Read the model definition and answer for the solid it produces. Units are mm, in the model's axes. A direction names the side the tool comes from. Give positions to 0.01 mm unless a question says otherwise; leave off trailing zeros. Write each loop counter-clockwise with the first axis right and the second up, starting at its lowest first coordinate (ties: lowest second). Pieces come first, ordered by that corner, then holes. Notation, with made-up numbers: (8.5, -10.5) -> (30.5, -10.5) arc R19 ccw to (30.5, 8.5) -> close; hole circle Ø9 at (-24, 65). An arc over 180 degrees is marked (long way). Answer as CSV lines item,"result". Start each with the question number.
1. Find the intervals of material crossed by line 1 (Y direction, x = 3, z = 78) (3 decimals); line 2 (Z direction, x = 1.5, y = 58.5) (3 decimals); line 3 (Y direction, x = 2.5, z = -12.5), in increasing order.
2. For a pull along Z with two mould halves and no side action, classify faces 3 (the cylindrical face through (3.219, 59.238, -17.206)), 4 (the flat face through (3, -43, -104.775)), 5 (the flat face through (3, -25, 53.975)), 6 (the flat face through (3, 69.85, 39)) as pulls with the +Z half, pulls with the -Z half, needs draft (parallel to the pull), parting line crosses it, or undercut.
3. The part is cut by section B-B, the plane y = -49. Determine the outline of the cut face in (x, z) (3 decimals).
4. The part is cut by section A-A, the plane x = 2.5. Give the number of separate pieces and of enclosed holes in the cut face, and give its area (3 significant figures).
5. A tool of negligible diameter and unlimited length cuts with its end or side. For faces 1 (the cylindrical face through (3.22, -103.11, 59.89)), 2 (the flat face through (3, 9.525, 80)), from which of +Z, -Z, +X, -X, +Y, -Y can it reach the whole face along a straight path? Write none if from no direction.
6. Given pin 1 (3 mm diameter, centred on y = 57.15, z = 60.325, fed in from +X); pin 2 (6.5 mm diameter, centred on y = 57.15, z = -15.875, fed in from +X); pin 3 (1.9 mm diameter, centred on x = 4, y = -13, fed in from +Z) (3 decimals); pin 4 (3 mm diameter, centred on x = 2.5, z = 67.5, fed in from +Y), each flat-ended and moving along its own axis, determine where each tip first touches the part or whether it passes through.
from build123d import *

# Parameters (mm, degrees)
SKETCH1_R               = 14.2875
BOSS_EXTRUDE1_DEPTH     = 6.35
SKETCH2_W               = 133.35
SKETCH2_H               = 44.45
CUT_EXTRUDE1_DEPTH      = 7.35
CUT_EXTRUDE2_DEPTH      = 7.35
BOSS_EXTRUDE2_DEPTH     = 6.35
SKETCH4_R               = 2.4765
CUT_EXTRUDE3_DEPTH      = 2.54
CUT_EXTRUDE3_DEPTH_BACK = 7.35


with BuildPart() as part:
    # Sketch1 → Boss-Extrude1 (new body)
    with BuildSketch(Plane(origin=(0, 0, 0), x_dir=(0, 0, -1), z_dir=(1, 0, 0))):
        Polygon((-104.775, -60.325), (-104.775, -114.3), (104.775, -114.3), (104.775, 114.3), (-104.775, 114.3), (-104.775, 9.525), (-53.975, 9.525), (-53.975, -60.325), align=None)
        with Locations((84.1375, 76.2)):
            Circle(SKETCH1_R, mode=Mode.SUBTRACT)
    extrude(amount=BOSS_EXTRUDE1_DEPTH)

    # Sketch2 → Cut-Extrude1 (cut, through all)
    with BuildSketch(Plane(origin=(6.35, 0, 0), x_dir=(0, 0, -1), z_dir=(1, 0, 0))):
        with Locations((-38.1, 92.075)):
            Rectangle(SKETCH2_W, SKETCH2_H)
    extrude(amount=-CUT_EXTRUDE1_DEPTH, mode=Mode.SUBTRACT)

    # Sketch3 → Cut-Extrude2 (cut, through all)
    with BuildSketch(Plane(origin=(6.35, 0, 0), x_dir=(0, 0, -1), z_dir=(1, 0, 0))):
        with BuildLine():
            Line((28.575, 114.3), (28.575, 69.85))
            Line((28.575, 69.85), (52.979857871, 100.782493632))
            ThreePointArc((52.979857871, 100.782493632), (61.948043641, 109.10479726), (73.025, 114.3))
            Line((73.025, 114.3), (28.575, 114.3))
        make_face()
        with BuildLine():
            Line((104.775, 114.3), (95.25, 114.3))
            ThreePointArc((95.25, 114.3), (100.150813391, 112.513516085), (104.775, 110.09972345))
            Line((104.775, 110.09972345), (104.775, 114.3))
        make_face()
    extrude(amount=-CUT_EXTRUDE2_DEPTH, mode=Mode.SUBTRACT)

    # Sketch3<3> → Boss-Extrude2 (add)
    with BuildSketch(Plane(origin=(6.35, 0, 0), x_dir=(0, 0, -1), z_dir=(1, 0, 0))):
        with BuildLine():
            ThreePointArc((119.268927195, 57.73705117), (113.070471033, 49.034197169), (104.775, 42.30027655))
            Line((104.775, 42.30027655), (104.775, 30.157905893))
            Line((104.775, 30.157905893), (119.268927195, 57.73705117))
        make_face()
        with BuildLine():
            Line((104.775, 110.09972345), (104.775, 42.30027655))
            ThreePointArc((104.775, 42.30027655), (113.070471033, 49.034197169), (119.268927195, 57.73705117))
            ThreePointArc((119.268927195, 57.73705117), (122.669150452, 66.691605303), (123.825, 76.2))
            ThreePointArc((123.825, 76.2), (118.736260364, 95.642824833), (104.775, 110.09972345))
        make_face()
        with BuildLine():
            ThreePointArc((95.25, 114.3), (84.1375, 115.8875), (73.025, 114.3))
            Line((73.025, 114.3), (95.25, 114.3))
        make_face()
    extrude(amount=-BOSS_EXTRUDE2_DEPTH)

    # Sketch4 → Cut-Extrude3 (cut, two sides)
    with BuildSketch(Plane(origin=(6.35, 0, 0), x_dir=(0, 0, -1), z_dir=(1, 0, 0))) as cut_extrude3_sk:
        with Locations((-60.325, 57.15)):
            Circle(SKETCH4_R)
        with Locations((15.875, 57.15)):
            Circle(SKETCH4_R)
        with Locations((92.075, -101.6)):
            Circle(SKETCH4_R)
        with Locations((-57.925, -101.6)):
            Circle(SKETCH4_R)
    extrude(amount=CUT_EXTRUDE3_DEPTH, mode=Mode.SUBTRACT)
    extrude(cut_extrude3_sk.sketch, amount=-CUT_EXTRUDE3_DEPTH_BACK, mode=Mode.SUBTRACT)


solid = part.part
Results found:
1,line 1,"y = -114.3 to -60.325, 9.525 to 69.85"
1,line 2,"z = -119.659 to -17.951, -13.799 to 58.249, 62.401 to 104.775"
1,line 3,"y = -114.3 to 69.85"
2,face 3,"undercut"
2,face 4,"pulls with the -Z half"
2,face 5,"pulls with the +Z half"
2,face 6,"needs draft"
3,outline,"(0, -104.775) -> (6.35, -104.775) -> (6.35, 53.975) -> (0, 53.975) -> close"
4,separate pieces,"1"
4,enclosed holes,"5"
4,area,"37,900 mm²"
5,face 1,"+X, -X"
5,face 2,"+Z, +X, -X"
6,pin 1,"passes through"
6,pin 2,"stops at x = 6.35"
6,pin 3,"stops at z = 53.975"
6,pin 4,"stops at y = 69.85"
